Verification items for this drawing (mm, ordinates from the low corner). A direction names the side the tool comes from. Give positions to 0.01 mm unless a question says otherwise; leave off trailing zeros. Order: outer loops, then holes, each group sorted by start corner. A loop starts at its lowest first (then second) coordinate and runs counter-clockwise, first axis right, second up.
(1) Access from +Z, -Z, +X, -X, +Y, -Y to the whole of each face (thin tool, end or side, straight path). Record for the marked faces 4, 5 and 6.
(2) Scan lines: L1, parallel to Z at x = 40, y = 13.25; L2, parallel to X at y = 18.25, z = 20; L3, parallel to Y at x = 5.5, z = 31. Record each from-to range of solid material in increasing order.
(3) Sectioned sample at D-D on z = 30. Record the cut outline in (x, y), plus the area to 3 significant figures.
(4) Mould release check, pull along X, two halves, no side actions. Record for the marked faces 1, 2 and 3: pulls with the +X half, pulls with the -X half, needs draft (parallel to the pull), parting line crosses it, or undercut.
(5) Sectioned sample at C-C on y = 11. Record the cut outline in (x, z), plus the area to 3 significant figures.
(6) Gauge pin test, flat ends, axial feed: pin 1 (8 mm diameter, centred on y = 17, z = 11.5, fed in from -X); pin 2 (5 mm diameter, centred on y = 16, z = 11, fed in from +X); pin 3 (3 mm diameter, centred on x = 37.5, z = 20.5, fed in from +Y). Record the tip position at first contact, or that the pin passes through.
(7) Sectioned sample at A-A on x = 40. Record the cut outline in (y, z), plus the area to 3 significant figures.
(8) Sectioned sample at B-B on z = 20. Record the cut outline in (x, y), plus the area to 3 significant figures.
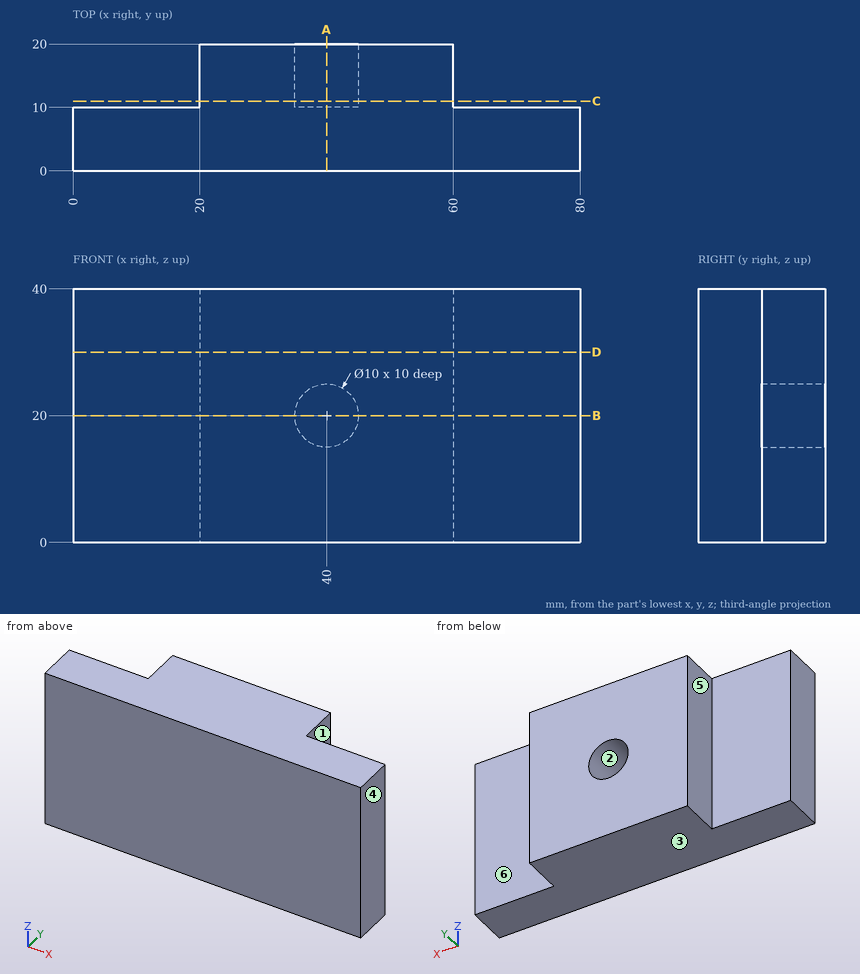
Ans:
1. face 4: +Z, -Z, +X, +Y, -Y
1. face 5: +Z, -Z, -X, +Y
1. face 6: +Z, -Z, +X, +Y
2. L1: z = 0 to 15, 25 to 40
2. L2: x = 20 to 35, 45 to 60
2. L3: y = 0 to 10
3. outline: (0, 0) - (80, 0) - (80, 10) - (60, 10) - (60, 20) - (20, 20) - (20, 10) - (0, 10) - close
3. area: 1,200 mm2
4. face 1: pulls with the +X half
4. face 2: undercut
4. face 3: needs draft
5. outline: (20, 0) - (60, 0) - (60, 40) - (20, 40) - close; hole circle Ø10 at (40, 20)
5. area: 1,520 mm2
6. pin 1: stops at x = 20
6. pin 2: stops at x = 60
6. pin 3: stops at y = 10
7. outline: (0, 0) - (20, 0) - (20, 15) - (10, 15) - (10, 25) - (20, 25) - (20, 40) - (0, 40) - close
7. area: 700 mm2
8. outline: (0, 0) - (80, 0) - (80, 10) - (60, 10) - (60, 20) - (45, 20) - (45, 10) - (35, 10) - (35, 20) - (20, 20) - (20, 10) - (0, 10) - close
8. area: 1,100 mm2
